Part model, mm, in its own coordinate system. Round coordinates to 2 decimals unless told otherwise and drop trailing zeros. Write each loop counter-clockwise with the first axis right and the second up, starting at its lowest first coordinate (ties: lowest second). Pieces come first, ordered by that corner, then holes. Notation, with made-up numbers: (-14.75, 76) -> (32.25, 76) arc R32 cw to (32.25, 108) -> close; hole circle Ø6 at (-5.5, -17). An arc over 180 degrees is marked (long way). Return JSON: item names as keys, results as strings. Group by question number.
(1) Mould opens along Y. For faces 1 (the flat face through (0, 0, 0)), 2 (the cylindrical face through (-30.235, -23.183, 37.656)), 3 (the flat face through (0, 0, 12.7)) say: +Y half, -Y half, draft (parallel to the pull), parting line (faces both ways), or undercut.
(2) Saw through at A-A (x = 0). List the corners of the cut face in (y, z), plus the area to 3 significant figures.
(3) Drop flat-ended pins along their axis: pin 1 Ø8 at (x, y) = (17.5, 13) entering from +Z; pin 2 Ø3 at (x, z) = (14.5, 67.5) entering from +Y; pin 3 Ø2 at (y, z) = (23.5, 36.5) entering from +X. Give the stop position or say it passes through.
(4) Drill centre lines: L1, parallel to Y at x = 0, z = 56; L2, parallel to X at y = -20, z = 16; L3, parallel to X at y = -29.5, z = 60.5. Where is each one in solid material? Low to high. Write a range as from..to.
(5) Saw through at C-C (z = 63.5). List the corners of the cut face in (x, y).
from build123d import *

# Parameters (mm, degrees)
F0_R     = 38.1
F1_DEPTH = 76.2
F2_R     = 6.35
F3_R     = 31.75
F4_DEPTH = 63.5
F5_R     = 6.35


with BuildPart() as f1:
    # F0 (on Top) → F1 (new body)
    with BuildSketch(Plane.XY):
        Circle(F0_R)
    extrude(amount=F1_DEPTH)

    # F2
    f2_edges = [f1.edges().sort_by_distance(p)[0] for p in [
        (-38.1, 0, 76.2),
        (-38.1, 0, 0),
    ]]
    fillet(f2_edges, radius=F2_R)

    # F3 (on face) → F4 (cut)
    with BuildSketch(Plane.XY.offset(76.2)):
        Circle(F3_R)
    extrude(amount=-F4_DEPTH, mode=Mode.SUBTRACT)

    # F5
    f5_edges = [f1.edges().sort_by_distance(p)[0] for p in [
        (-31.75, 0, 12.7),
    ]]
    fillet(f5_edges, radius=F5_R)


solid = f1.part
Computed values:
{
 "1": {"face 1": "draft", "face 2": "parting line", "face 3": "undercut"},
 "2": {"outline": "(-38.1, 6.35) arc R6.35 ccw to (-31.75, 0) -> (31.75, 0) arc R6.35 ccw to (38.1, 6.35) -> (38.1, 69.85) arc R6.35 ccw to (31.75, 76.2) -> (31.75, 19.05) arc R6.35 cw to (25.4, 12.7) -> (-25.4, 12.7) arc R6.35 cw to (-31.75, 19.05) -> (-31.75, 76.2) arc R6.35 ccw to (-38.1, 69.85) -> close", "area": "1,760 mm2"},
 "3": {"pin 1": "z = 12.71", "pin 2": "y = 35.81", "pin 3": "x = 30.75"},
 "4": {"L1": "-38.1..-31.75, 31.75..38.1", "L2": "-32.43..-23.65, 23.65..32.43", "L3": "-24.11..-11.74, 11.74..24.11"},
 "5": {"outline": "circle Ø76.2 at (0, 0); hole circle Ø63.5 at (0, 0)"}
}
